```python
from build123d import *

# Parameters (mm, degrees)
CUT_EXTRUDE_1_DEPTH = 1.5
FILLET_1_R          = 0.3


with BuildPart() as part:
    # 草图1 → 旋转1 (revolve)
    with BuildSketch(Plane(origin=(0, 0, 0), x_dir=(0, 0, -1), z_dir=(1, 0, 0)), mode=Mode.PRIVATE) as revolve_1_sk:
        Polygon((-7.5, 0), (-7.5, 3), (-7, 3), (-5.5, 1.5), (7.2, 1.5), (7.5, 1.2), (7.5, 0), align=None)
    revolve(revolve_1_sk.sketch.rotate(Axis((0, 0, -7.5), (0, 0, 1)), 90), axis=Axis((0, 0, -7.5), (0, 0, 1)))

    # 草图2 → 切除-拉伸1 (cut)
    with BuildSketch(Plane.XY.offset(7.5)):
        Polygon((1.154700538, 0), (0.577350269, 1), (-0.577350269, 1), (-1.154700538, 0), (-0.577350269, -1), (0.577350269, -1), align=None)
    extrude(amount=-CUT_EXTRUDE_1_DEPTH, mode=Mode.SUBTRACT)

    # 圆角1
    fillet_1_edges = [part.edges().sort_by_distance(p)[0] for p in [
        (3, 0, 7.5),
    ]]
    fillet(fillet_1_edges, radius=FILLET_1_R)


solid = part.part
```
Read the model definition and answer for the solid it produces. Units are mm, in the model's axes. A direction names the side the tool comes from. Coordinates: 2 decimals unless noted, no trailing zeros. Loops run counter-clockwise (first coordinate to the right, second up) from the corner with the lowest first, then second, coordinate; pieces in that order, holes last. Notation, with made-up numbers: (59.25, -32.75) - (73.25, -32.75) arc R25 ccw to (73.25, -13.75) - close; hole circle Ø5 at (76.25, -40). An arc over 180 degrees is marked (long way). Answer in a Markdown table with one row per item.
1. Determine the mould class of faces 1 (the face through (-0.86, 0.51, 6.76)), 2 (the face through (0, 1, 7)), 3 (the face through (0, 0, -7.5)), 4 (the face through (0, 2, 6)) for opening direction Y: +Y half, -Y half, draft (parallel to the pull), parting line (faces both ways), or undercut.
Conclusion:
| item | result |
|---|---|
| face 1 | undercut |
| face 2 | undercut |
| face 3 | draft |
| face 4 | parting line |
2. Given pin 1 (3 mm diameter, centred on x = -1.5, z = 3, fed in from -Y); pin 2 (1.5 mm diameter, centred on y = 1, z = 3.5, fed in from +X); pin 3 (0.6 mm diameter, centred on x = 0.5, y = 0, fed in from +Z); pin 4 (1 mm diameter, centred on x = 2.5, z = 5, fed in from -Y), each flat-ended and moving along its own axis, determine where each tip first touches the part or whether it passes through.
Conclusion:
| item | result |
|---|---|
| pin 1 | stops at y = -1.5 |
| pin 2 | stops at x = 1.48 |
| pin 3 | stops at z = 6 |
| pin 4 | passes through |
3. Which of the six approach directions +Z, -Z, +X, -X, +Y, -Y give full straight-line access (tool end or side, diameter ignored) to faces 5 (the face through (0, 1.2, 7.5)), 6 (the face through (-1.43, -0.45, -0.94)), 7 (the face through (0, -1, 7))?
Conclusion:
| item | result |
|---|---|
| face 5 | +Z, +X, -X, +Y, -Y |
| face 6 | -Z |
| face 7 | +Z |
4. Find section A-A, the plane x = 0. Write down the section's boundary in (y, z), then the cut area to 3 significant figures.
Conclusion:
| item | result |
|---|---|
| outline | (-3, 7) - (-1.5, 5.5) - (-1.5, -7.2) - (-1.2, -7.5) - (1.2, -7.5) - (1.5, -7.2) - (1.5, 5.5) - (3, 7) - (3, 7.2) arc R0.3 ccw to (2.7, 7.5) - (1, 7.5) - (1, 6) - (-1, 6) - (-1, 7.5) - (-2.7, 7.5) arc R0.3 ccw to (-3, 7.2) - close |
| area | 45.6 mm² |
5. Find section B-B, the plane z = 0. Write down the section's boundary in (x, y), then the cut area to 3 significant figures.
Conclusion:
| item | result |
|---|---|
| outline | circle Ø3 at (0, 0) |
| area | 7.07 mm² |
6. Straight lines are drawn through the part: line 1 (Z direction, x = -0.25, y = 0.5); line 2 (X direction, y = -0.5, z = -2.75); line 3 (Y direction, x = -0.25, z = -1.25). For each, find the intervals that lie inside material, in ascending order.
Conclusion:
| item | result |
|---|---|
| line 1 | z = -7.5 to 6 |
| line 2 | x = -1.41 to 1.41 |
| line 3 | y = -1.48 to 1.48 |
